```python
from build123d import *

# Parameters (mm, degrees)
SKETCH1_W                       = 30
SKETCH1_H                       = 194.2
SKETCH1_H_2                     = 27
SKETCH1_H_3                     = 261.4
EXTRUDE1_DEPTH                  = 15
FILLET1_R                       = 10
EXTRUDE2_DEPTH                  = 10
SKETCH3_W                       = 80
SKETCH3_H                       = 25
EXTRUDE3_DEPTH                  = 30
SKETCH5_W                       = 70
SKETCH5_H                       = 20
EXTRUDE4_DEPTH                  = 24
FILLET2_R                       = 10
EXTRUDE5_REACH                  = 432.349
SKETCH6_R                       = 4.029178008
SKETCH7_W                       = 30
SKETCH7_H                       = 263.372286267
EXTRUDE6_DEPTH                  = 427.91910061
EXTRUDE7_DEPTH                  = 100
SKETCH9_W                       = 30
SKETCH9_H                       = 136.58118173
EXTRUDE8_DEPTH                  = 10
F_1_4_0_25_DIAMETER_HOLE1_D     = 6.35
F_1_4_0_25_DIAMETER_HOLE1_DEPTH = 10
F_1_4_0_25_DIAMETER_HOLE1_TIP   = 1.907732465
EXTRUDE10_DEPTH                 = 439.560051151
EXTRUDE10_DEPTH_BACK            = 439.560051151
SKETCH11_W                      = 9.397052114
SKETCH11_H                      = 50.5
SKETCH12_R                      = 10
EXTRUDE11_DEPTH                 = 10


with BuildPart() as part:
    # Sketch1 → Extrude1 (new body)
    with BuildSketch(Plane.XY):
        with Locations((15, 322.665015772)):
            Rectangle(SKETCH1_W, SKETCH1_H)
        with BuildLine():
            Line((30, 225.565015772), (30, 198.565015772))
            Line((30, 198.565015772), (50, 198.565015772))
            ThreePointArc((50, 198.565015772), (63.5, 212.065015772), (50, 225.565015772))
            Line((50, 225.565015772), (30, 225.565015772))
        make_face()
        with Locations((15, 212.065015772)):
            Rectangle(SKETCH1_W, SKETCH1_H_2)
        with BuildLine():
            Line((-20, 198.565015772), (0, 198.565015772))
            Line((0, 198.565015772), (0, 225.565015772))
            Line((0, 225.565015772), (-20, 225.565015772))
            ThreePointArc((-20, 225.565015772), (-33.5, 212.065015772), (-20, 198.565015772))
        make_face()
        with Locations((15, 67.865015772)):
            Rectangle(SKETCH1_W, SKETCH1_H_3)
    extrude(amount=EXTRUDE1_DEPTH)

    # Fillet1
    fillet1_edges = [part.edges().sort_by_distance(p)[0] for p in [
        (0, 419.765015772, 7.5),
        (30, 419.765015772, 7.5),
        (30, -62.834984228, 7.5),
        (0, -62.834984228, 7.5),
    ]]
    fillet(fillet1_edges, radius=FILLET1_R)

    # Sketch2 → Extrude2 (cut)
    with BuildSketch(Plane(origin=(0, 0, 0), x_dir=(-1, 0, 0), z_dir=(0, 0, -1))):
        with BuildLine():
            Line((-50, 225.565015772), (-30, 225.565015772))
            Line((-30, 225.565015772), (-30, 198.565015772))
            Line((-30, 198.565015772), (-50, 198.565015772))
            ThreePointArc((-50, 198.565015772), (-63.5, 212.065015772), (-50, 225.565015772))
        make_face()
        with BuildLine():
            Line((0, 198.565015772), (20, 198.565015772))
            ThreePointArc((20, 198.565015772), (33.5, 212.065015772), (20, 225.565015772))
            Line((20, 225.565015772), (0, 225.565015772))
            Line((0, 225.565015772), (0, 198.565015772))
        make_face()
    extrude(amount=-EXTRUDE2_DEPTH, mode=Mode.SUBTRACT)

    # Sketch3 → Extrude3 (add)
    with BuildSketch(Plane.XY.offset(15)):
        with Locations((15, 407.265015772)):
            Rectangle(SKETCH3_W, SKETCH3_H)
    extrude(amount=EXTRUDE3_DEPTH)

    # Sketch5 → Extrude4 (cut)
    with BuildSketch(Plane.XY.offset(45)):
        with Locations((15, 409.765015772)):
            Rectangle(SKETCH5_W, SKETCH5_H)
    extrude(amount=-EXTRUDE4_DEPTH, mode=Mode.SUBTRACT)

    # Fillet2
    fillet2_edges = [part.edges().sort_by_distance(p)[0] for p in [
        (52.5, 419.765015772, 45),
        (-22.5, 419.765015772, 45),
    ]]
    fillet(fillet2_edges, radius=FILLET2_R)

    # Sketch6 → Extrude5 (add, up to next)
    with BuildSketch(Plane.ZY.offset(-50), mode=Mode.PRIVATE) as extrude5_sk1:
        with Locations(Location((35, 413.847695375, 0), (0, 0, 180))):
            Circle(SKETCH6_R)
    extrude5_tool1 = extrude(extrude5_sk1.sketch, amount=EXTRUDE5_REACH, mode=Mode.PRIVATE) - part.part
    add(extrude5_tool1.solids().sort_by_distance((50, 413.847695, 35))[0])

    # Sketch7 → Extrude6 (cut, through all)
    with BuildSketch(Plane(origin=(0, 0, 0), x_dir=(-1, 0, 0), z_dir=(0, 0, -1))):
        with Locations((-15, 66.878872639)):
            Rectangle(SKETCH7_W, SKETCH7_H)
    extrude(amount=-EXTRUDE6_DEPTH, mode=Mode.SUBTRACT)

    # Sketch8 → Extrude7 (add)
    with BuildSketch(Plane(origin=(0, 0, 0), x_dir=(-1, 0, 0), z_dir=(0, 0, -1))):
        Polygon((-30, 198.565015772), (0, 198.565015772), (0, 225.565015772), (-5, 225.565015772), (-5, 203.565015772), (-25, 203.565015772), (-25, 225.565015772), (-30, 225.565015772), align=None)
    extrude(amount=EXTRUDE7_DEPTH)

    # Sketch9 → Extrude8 (add)
    with BuildSketch(Plane(origin=(0, 0, -100), x_dir=(-1, 0, 0), z_dir=(0, 0, -1))):
        with Locations((-15, 157.274424907)):
            Rectangle(SKETCH9_W, SKETCH9_H)
    extrude(amount=EXTRUDE8_DEPTH)

    # 1/4 (0.25) Diameter Hole1
    with Locations(Plane(origin=(-20, 212.065015772, 10), x_dir=(-1, 0, 0), z_dir=(0, 0, -1))):
        with Locations((0, 0), (-70, 0)):
            Hole(F_1_4_0_25_DIAMETER_HOLE1_D / 2, depth=F_1_4_0_25_DIAMETER_HOLE1_DEPTH)
            with Locations((0, 0, -(F_1_4_0_25_DIAMETER_HOLE1_DEPTH + F_1_4_0_25_DIAMETER_HOLE1_TIP / 2))):  # 118° drill point
                Cone(0, F_1_4_0_25_DIAMETER_HOLE1_D / 2, F_1_4_0_25_DIAMETER_HOLE1_TIP, mode=Mode.SUBTRACT)

    # Sketch11 → Extrude10 (cut, two sides: drawn at the far end of the back side and taken through both)
    with BuildSketch(Plane(origin=(30, 0, 0), x_dir=(0, 0, -1), z_dir=(1, 0, 0)).offset(-EXTRUDE10_DEPTH_BACK)):
        with Locations((-10.301473943, 223.815015772)):
            Rectangle(SKETCH11_W, SKETCH11_H)
    extrude(amount=EXTRUDE10_DEPTH + EXTRUDE10_DEPTH_BACK, mode=Mode.SUBTRACT)

    # Sketch12 → Extrude11 (add)
    with BuildSketch(Plane.XY.offset(5.602947886)):
        with Locations(Location((14.080124671, 212.060594596, 0), (0, 0, 90))):
            Circle(SKETCH12_R)
    extrude(amount=EXTRUDE11_DEPTH)


solid = part.part
```
Could you check a few things on this model? Use its own coordinates, in mm. A direction names the side the tool comes from. Coordinates: 2 decimals unless noted, no trailing zeros. Loops run counter-clockwise (first coordinate to the right, second up) from the corner with the lowest first, then second, coordinate; pieces in that order, holes last.
1) Imagine slicing it at D-D (y = 330.5). List the corners of the cut face in (x, z) for me, and give its area (3 significant figures).
Reported:
outline: (0, 0) - (30, 0) - (30, 15) - (0, 15) - close
area: 450 mm2
2) Which directions (+Z, -Z, +X, -X, +Y, -Y) give clear straight access to the entire face, cutting with the end or side of a thin tool? Please do faces 1 (the face through (14, 212, 15.603)), 2 (the face through (-20, 410, 33)), 3 (the face through (15, 203.565, -49)).
Reported:
face 1: +Z, +X, -X, -Y
face 2: none
face 3: +Y
3) Imagine slicing it at B-B (z = -63.5). List the corners of the cut face in (x, y) for me, and give its area (3 significant figures).
Reported:
outline: (0, 198.57) - (30, 198.57) - (30, 225.57) - (25, 225.57) - (25, 203.57) - (5, 203.57) - (5, 225.57) - (0, 225.57) - close
area: 370 mm2
4) Will these pins go through, and if not, where does the flat tip stop? pin 1 Ø3 at (x, y) = (25.5, 236) entering from +Z; pin 2 Ø3 at (x, z) = (21.5, 12.5) entering from -Y; pin 3 Ø9 at (x, y) = (18.5, 343) entering from +Z.
Reported:
pin 1: stops at z = 5.6
pin 2: stops at y = 204
pin 3: stops at z = 15
5) Please list where these lines run through material, in increasing order: line 1 along Z through (x, y) = (25, 120); line 2 along Z through (x, y) = (27, 220); line 3 along Y through (x, z) = (35.5, 16).
Reported:
line 1: z = -110 to -100
line 2: z = -110 to 5.6
line 3: y = 394.77 to 419.77
6) Thinking about a two-plate mould opening in Y: for faces 4 (the face through (15.5, 417.4, 33.1)), 5 (the face through (15, 410, 21)), 6 (the face through (15, 198.565, -46)), which applies, released by +Y, released by -Y, zero draft, split by the parting line, or undercut?
Reported:
face 4: undercut
face 5: zero draft
face 6: released by -Y
7) Imagine slicing it at C-C (x = 44.5). List the corners of the cut face in (y, z) for me, and give its area (3 significant figures).
Reported:
outline: (394.77, 15) - (419.77, 15) - (419.77, 21) - (399.77, 21) - (399.77, 45) - (394.77, 45) - close; circle Ø8.06 at (413.85, 35)
area: 321 mm2
8) Imagine slicing it at A-A (z = 9). List the corners of the cut face in (x, y) for me, and give its area (3 significant figures).
Reported:
outline: (0, 249.07) - (30, 249.07) - (30, 409.77) arc R10 ccw to (20, 419.77) - (10, 419.77) arc R10 ccw to (0, 409.77) - close; circle Ø20 at (14.08, 212.06)
area: 5,390 mm2
